The drawing under review shows one solid part. Ordinate dimensions are in mm from its lowest x, y, z. Round coordinates to 2 decimals unless told otherwise and drop trailing zeros. Write each loop counter-clockwise with the first axis right and the second up, starting at its lowest first coordinate (ties: lowest second). Pieces come first, ordered by that corner, then holes. Notation, with made-up numbers: (61, 77) -> (97, 77) arc R19 cw to (97, 111) -> close; hole circle Ø3 at (83, 61). An arc over 180 degrees is marked (long way). Answer in a Markdown table with one row per item. Add a question column.
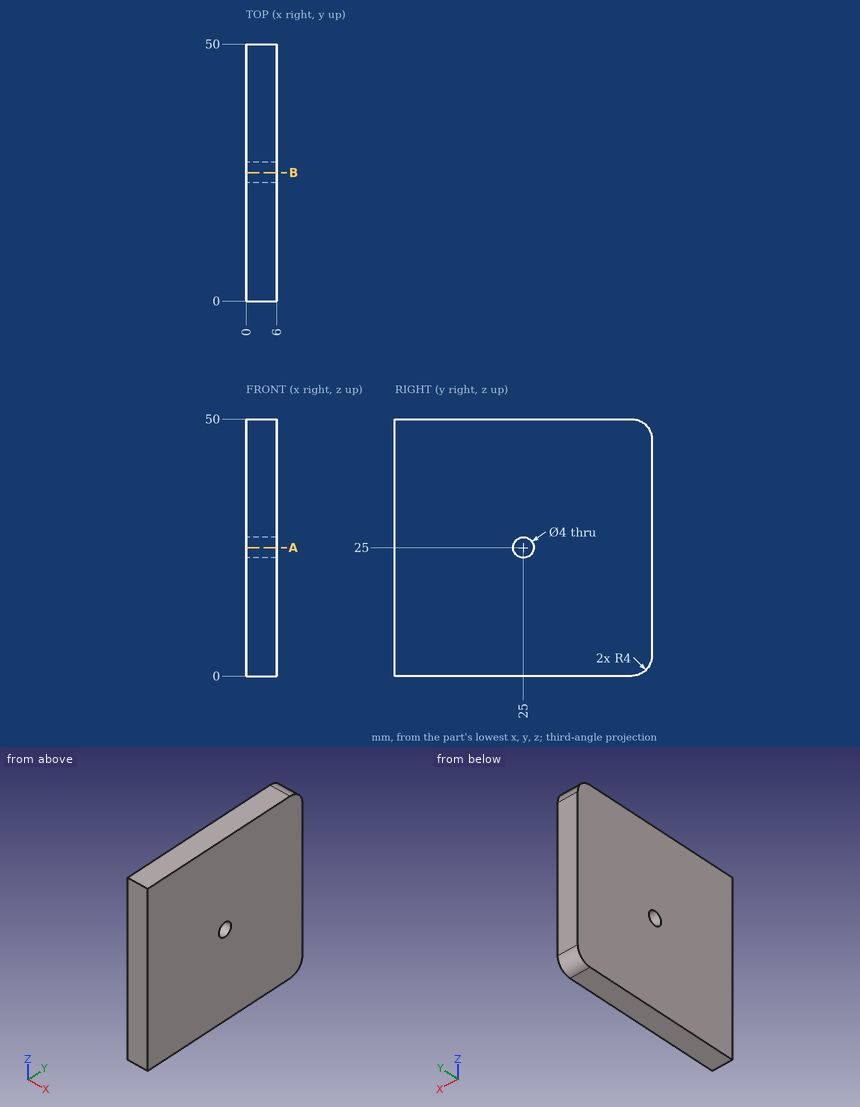
1. For L1, parallel to Y at x = 4, z = 25; L2, parallel to Y at x = 1.8, z = 48.5, list the stretches that pass through material, from the lowest coordinate up.
2. Add section A-A on z = 25. Write out the cut boundary in (x, y), plus the area to 3 significant figures.
Filled in:
| question | item | result |
|---|---|---|
| 1 | L1 | 0 to 23, 27 to 50 |
| 1 | L2 | 0 to 49.12 |
| 2 | outline | (0, 0) -> (6, 0) -> (6, 23) -> (0, 23) -> close; (0, 27) -> (6, 27) -> (6, 50) -> (0, 50) -> close |
| 2 | area | 276 mm² |
